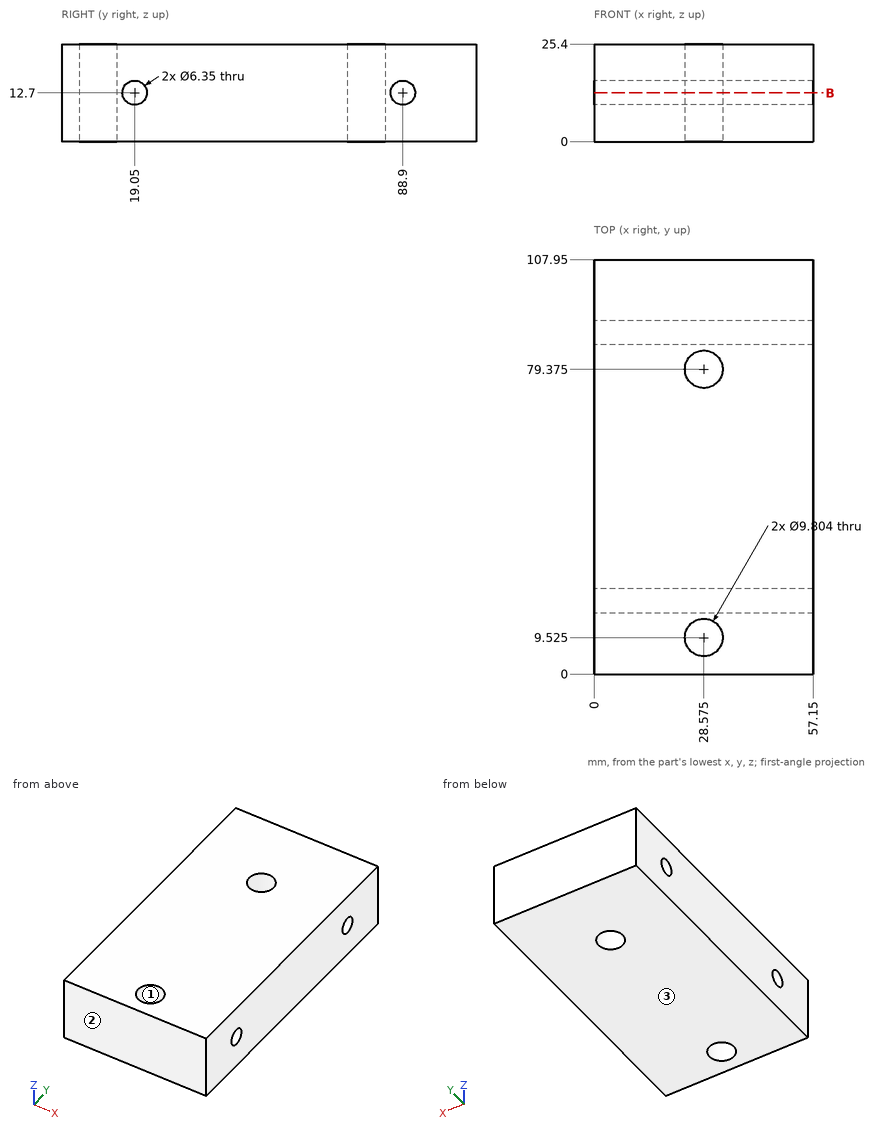
Drawing for the job (mm, zero at the part's lowest x, y, z). Coordinates: 2 decimals unless noted, no trailing zeros. One line per item, written item: value. Start each with the question number.
1) Pull direction Y, two halves, no side cores. Call the marked faces 1, 2 and 3: +Y half, -Y half, draft (parallel to the pull), parting line (faces both ways), or undercut.
2) Probe probe 1 along Y at (x, z) = (28.5, 17); probe 2 along Y at (x, z) = (27, 20.25); probe 3 along Z at (x, y) = (36, 19) (1 decimal). List the from-to ranges inside material, lowest first.
3) Slice it at B-B on z = 12.7. Count the separate pieces of the cut face and the enclosed holes in it, then the cut area to 3 significant figures.
Answers follow:
1. face 1: undercut
1. face 2: -Y half
1. face 3: draft
2. probe 1: 0 to 4.62, 14.43 to 74.47, 84.28 to 107.95
2. probe 2: 0 to 4.88, 14.17 to 74.73, 84.02 to 107.95
2. probe 3: 0 to 9.5, 15.9 to 25.4
3. separate pieces: 3
3. enclosed holes: 2
3. area: 5,290 mm2
